Can you work these out from the model? Positions are in its coordinate system, mm. A direction names the side the tool comes from. Coordinates: 2 decimals unless noted, no trailing zeros. Loops run counter-clockwise (first coordinate to the right, second up) from the corner with the lowest first, then second, coordinate; pieces in that order, holes last. Notation, with made-up numbers: (3.25, 11.5) -> (22.25, 11.5) arc R18 cw to (22.25, 27.5) -> close; hole circle Ø9 at (47, 55). An arc over 180 degrees is marked (long way). Put each result on its own line as item: value. Start each with the question number.
Item 1: We'd pull the mould along X, two halves only. Please class faces 1 (the cylindrical face through (-11.9, -24.5, 1)), 2 (the flat face through (0, -27.5, 1)), 3 (the flat face through (-18.75, 0, 6)), 4 (the cylindrical face through (12, 21.5, 1)): pulls with the +X half, pulls with the -X half, needs draft (parallel to the pull), parting line crosses it, or undercut.
Item 2: Please list where these lines run through material, in increasing order: L1, parallel to Y at x = -11.95, z = 1.6; L2, parallel to X at y = 23, z = 1.4; L3, parallel to Y at x = 4.5, z = 2.5. Write a range as from..to.
Item 3: Will these pins go through, and if not, where does the flat tip stop? P1, Ø2.5, axis at x = 1.5, y = -22.5, coming from the +Z side; P2, Ø1.8, axis at x = -11.95, y = 23, coming from the -Z side; P3, Ø1.5, axis at x = -0.5, z = 5, coming from the +Y side.
Item 4: If we section it at B-B on y = 23: Please give me the cut outline in (x, z).
Item 5: For faces 5 (the flat face through (0, 0, 0)), 6 (the flat face through (0, 18.75, 7)), 7 (the flat face through (0, -18.75, 7)), which set-ups out of +Z, -Z, +X, -X, +Y, -Y let a thin tool reach every point of the face, with its end or its side?
Item 6: If we section it at A-A on x = -11.95: Please give me the cut outline in (y, z).
Item 7: If we section it at C-C on x = -3: Please give me the cut outline in (y, z).
Item 8: If we section it at D-D on z = 11.5: Please give me the cut outline in (x, y), plus the area to 3 significant figures.
Solid Edge part; units mm, degrees
sketch "Sketch1" plane through (0, 0, 0) normal (0, 0, 1) x (1, 0, 0)
  line L0 (-18.75, -27.5) -> (18.75, -27.5)
  line L1 (18.75, -27.5) -> (18.75, 27.5)
  line L2 (18.75, 27.5) -> (-18.75, 27.5)
  line L3 (-18.75, 27.5) -> (-18.75, -27.5)
  dimension "D1" = 18.75
  dimension "D2" = 18.75
extrude "Protrusion1" add sketch "Sketch1" along normal blind 2
sketch "Sketch2" plane through (0, 0, 2) normal (0, 0, 1) x (1, 0, 0)
  line L0 (-18.75, -18.75) -> (18.75, -18.75)
  line L1 (18.75, -18.75) -> (18.75, 18.75)
  line L2 (18.75, 18.75) -> (-18.75, 18.75)
  line L3 (-18.75, 18.75) -> (-18.75, -18.75)
  dimension "D1" = 18.75
extrude "Extrusionsausprägung_2" add sketch "Sketch2" along normal blind 10.5
hole "Bohrung_1" at (-11.95, 23, 0) direction (0, 0, 1) diameter 3 end up to next
hole "Hole1" at (-11.95, -23, 0) direction (0, 0, 1) diameter 3 end up to next
hole "Hole2" at (11.95, -23, 0) direction (0, 0, 1) diameter 3 end up to next
hole "Hole3" at (11.95, 23, 0) direction (0, 0, 1) diameter 3 end up to next
Solutions:
1. face 1: undercut
1. face 2: needs draft
1. face 3: pulls with the -X half
1. face 4: undercut
2. L1: -27.5..-24.5, -21.5..21.5, 24.5..27.5
2. L2: -18.75..-13.45, -10.45..10.45, 13.45..18.75
2. L3: -18.75..18.75
3. P1: z = 2
3. P2: through
3. P3: y = 18.75
4. outline: (-18.75, 0) -> (-13.45, 0) -> (-13.45, 2) -> (-18.75, 2) -> close; (-10.45, 0) -> (10.45, 0) -> (10.45, 2) -> (-10.45, 2) -> close; (13.45, 0) -> (18.75, 0) -> (18.75, 2) -> (13.45, 2) -> close
5. face 5: -Z, +X, -X, +Y, -Y
5. face 6: +Z, +X, -X, +Y
5. face 7: +Z, +X, -X, -Y
6. outline: (-27.5, 0) -> (-24.5, 0) -> (-24.5, 2) -> (-27.5, 2) -> close; (-21.5, 0) -> (21.5, 0) -> (21.5, 2) -> (18.75, 2) -> (18.75, 12.5) -> (-18.75, 12.5) -> (-18.75, 2) -> (-21.5, 2) -> close; (24.5, 0) -> (27.5, 0) -> (27.5, 2) -> (24.5, 2) -> close
7. outline: (-27.5, 0) -> (27.5, 0) -> (27.5, 2) -> (18.75, 2) -> (18.75, 12.5) -> (-18.75, 12.5) -> (-18.75, 2) -> (-27.5, 2) -> close
8. outline: (-18.75, -18.75) -> (18.75, -18.75) -> (18.75, 18.75) -> (-18.75, 18.75) -> close
8. area: 1,410 mm^2
